Could you check a few things on this model? Use its own coordinates, in mm. Face numbers are marked on the shaded views. A direction names the side the tool comes from. Round coordinates to 2 decimals unless told otherwise and drop trailing zeros. Write each loop counter-clockwise with the first axis right and the second up, starting at its lowest first coordinate (ties: lowest second). Pieces come first, ordered by that corner, then holes. Notation, with made-up numbers: (68.5, -34) - (103.5, -34) arc R13 ccw to (103.5, -14) - close; hole circle Ø7 at (83.5, 16.5). An arc over 180 degrees is marked (long way). Put each result on its own line as item: value.
from build123d import *

# Parameters (mm, degrees)
SKETCH1_W           = 70
SKETCH1_H           = 55.65
BOSS_EXTRUDE1_DEPTH = 16.83
BOSS_EXTRUDE2_START = 16.83
SKETCH2_W           = 30.33
SKETCH2_H           = 30
BOSS_EXTRUDE2_DEPTH = 6.35
SKETCH3_R           = 14.055
BOSS_EXTRUDE3_DEPTH = 6.35
SKETCH4_R           = 14.055
CUT_EXTRUDE1_DEPTH  = 6.35
BOSS_EXTRUDE4_START = -35
SKETCH5_W           = 9.44
SKETCH5_H           = 4.86
BOSS_EXTRUDE4_DEPTH = 6.76
SKETCH6_R           = 1.7
BOSS_EXTRUDE5_DEPTH = 4
FILLET1_R           = 3
SKETCH7_R           = 7.14
BOSS_EXTRUDE6_DEPTH = 6.35
BOSS_EXTRUDE7_DEPTH = 4.35
FILLET3_R           = 3.5
CIRPATTERN11_COUNT  = 7
FILLET4_R           = 3.5


with BuildPart() as part:
    # Sketch1 → Boss-Extrude1 (new body)
    with BuildSketch(Plane(origin=(0, 0, 0), x_dir=(1, 0, 0), z_dir=(0, 1, 0))):
        Rectangle(SKETCH1_W, SKETCH1_H)
    extrude(amount=BOSS_EXTRUDE1_DEPTH)

    # Sketch2 → Boss-Extrude2 (add)
    with BuildSketch(Plane(origin=(0, 0, 0), x_dir=(1, 0, 0), z_dir=(0, 1, 0)).offset(BOSS_EXTRUDE2_START)):
        Rectangle(SKETCH2_W, SKETCH2_H)
    extrude(amount=BOSS_EXTRUDE2_DEPTH)

    # Sketch3 → Boss-Extrude3 (add)
    with BuildSketch(Plane(origin=(0, 23.18, 0), x_dir=(1, 0, 0), z_dir=(0, 1, 0))):
        Circle(SKETCH3_R)
    extrude(amount=-BOSS_EXTRUDE3_DEPTH)

    # Sketch4 → Cut-Extrude1 (cut)
    with BuildSketch(Plane(origin=(0, 23.18, 0), x_dir=(1, 0, 0), z_dir=(0, 1, 0))):
        with Locations(Location((0, 0, 0), (0, 0, 270))):
            Circle(SKETCH4_R)
    extrude(amount=-CUT_EXTRUDE1_DEPTH, mode=Mode.SUBTRACT)

    # Sketch5 → Boss-Extrude4 (add)
    with BuildSketch(Plane(origin=(0, 0, 0), x_dir=(0, 0, -1), z_dir=(1, 0, 0)).offset(BOSS_EXTRUDE4_START)):
        with Locations((18.775, 6.43)):
            Rectangle(SKETCH5_W, SKETCH5_H)
    extrude(amount=-BOSS_EXTRUDE4_DEPTH)

    # Sketch6 → Boss-Extrude5 (add)
    with BuildSketch(Plane(origin=(35, 0, 0), x_dir=(0, 0, -1), z_dir=(1, 0, 0))):
        with Locations(Location((-19.125364984, 11.29, 0), (0, 0, 180))):
            Circle(SKETCH6_R)
        with Locations(Location((-9.475364984, 11.29, 0), (0, 0, 180))):
            Circle(SKETCH6_R)
    extrude(amount=BOSS_EXTRUDE5_DEPTH)

    # Fillet1
    fillet1_edges = [part.edges().sort_by_distance(p)[0] for p in [
        (-35, 8.415, -27.825),
        (35, 8.415, -27.825),
        (35, 8.415, 27.825),
        (-35, 8.415, 27.825),
    ]]
    fillet(fillet1_edges, radius=FILLET1_R)

    # Sketch7 → Boss-Extrude6 (add)
    with BuildSketch(Plane(origin=(0, 16.83, 0), x_dir=(1, 0, 0), z_dir=(0, 1, 0))):
        with Locations(Location((0, 0, 0), (0, 0, 270))):
            Circle(SKETCH7_R)
    extrude(amount=BOSS_EXTRUDE6_DEPTH)

    # Sketch11 → Boss-Extrude7 (add)
    with BuildSketch(Plane(origin=(0, 16.83, 0), x_dir=(1, 0, 0), z_dir=(0, 1, 0))):
        with BuildLine():
            ThreePointArc((7.116145586, -0.583156929), (6.803943672, -2.164705639), (6.144899887, -3.635905029))
            ThreePointArc((6.144899887, -3.635905029), (11.187164412, -1.887909247), (13.51656418, 2.913529862))
            ThreePointArc((13.51656418, 2.913529862), (10.713284894, 0.438636341), (7.116145586, -0.583156929))
        make_face()
    boss_extrude7 = extrude(amount=BOSS_EXTRUDE7_DEPTH)

    # Fillet3
    # the kernel refuses this fillet: 3.5 mm, written as the material it takes off along each edge
    with BuildSketch(Plane(origin=(6.556014588, 21.18, -3.324644563), x_dir=(-0.9673093233437143, 0, 0.25359943409307006), z_dir=(-0.25359943409307006, 0, -0.9673093233437143))) as fillet3_piece_1_section:
        with BuildLine():
            CenterArc((6.972679966 - FILLET3_R, -FILLET3_R), FILLET3_R, 0, 90)
            Line((6.972679966 - FILLET3_R, 0), (6.972679966, 0))
            Line((6.972679966, 0), (6.972679966, -FILLET3_R))
        make_face()
    fillet3_piece_1 = revolve(axis=Axis((6.556014588, 21.18, -3.324644563), (0, 1, 0)), revolution_arc=233.858448906, mode=Mode.PRIVATE)
    fillet3_piece_1 = fillet3_piece_1 - Plane(origin=(0, 20.294110175, 0), x_dir=(0, 0, 1), z_dir=(0, -1, 0)) * Cylinder(7.14, 28, mode=Mode.PRIVATE)
    fillet3_piece_1 = fillet3_piece_1 - Plane(origin=(6.664387144, 20.294110175, -7.849834998), x_dir=(0.8113805957786566, 0, 0.5845182022776301), z_dir=(0, -1, 0)) * Cylinder(8.445083689, 28, mode=Mode.PRIVATE)
    add(fillet3_piece_1, mode=Mode.SUBTRACT)

    # CirPattern11: Boss-Extrude7 ×7 about axis
    cirpattern11_axis = Axis((0, 0, 0), (0, 1, 0))
    for i in range(1, CIRPATTERN11_COUNT):
        add(boss_extrude7.rotate(cirpattern11_axis, i * 360 / CIRPATTERN11_COUNT))

    # Fillet4
    # the kernel refuses this fillet: 3.5 mm, written as the material it takes off along each edge
    with BuildSketch(Plane(origin=(6.686920024, 21.18, 3.052816625), x_dir=(-0.8013795198577165, 0, -0.5981562213607877), z_dir=(0.5981562213607877, 0, -0.8013795198577165))) as fillet4_piece_1_section:
        with BuildLine():
            CenterArc((6.972679966 - FILLET4_R, -FILLET4_R), FILLET4_R, 0, 90)
            Line((6.972679966 - FILLET4_R, 0), (6.972679966, 0))
            Line((6.972679966, 0), (6.972679966, -FILLET4_R))
        make_face()
    fillet4_piece_1 = revolve(axis=Axis((6.686920024, 21.18, 3.052816625), (0, 1, 0)), revolution_arc=233.858448906, mode=Mode.PRIVATE)
    fillet4_piece_1 = fillet4_piece_1 - Plane(origin=(0, 20.294110175, 0), x_dir=(0, 0, 1), z_dir=(0, -1, 0)) * Cylinder(7.14, 28, mode=Mode.PRIVATE)
    fillet4_piece_1 = fillet4_piece_1 - Plane(origin=(10.292425554, 20.294110175, 0.316135614), x_dir=(0.04889279427778842, 0, 0.998804032164323), z_dir=(0, -1, 0)) * Cylinder(8.445083689, 28, mode=Mode.PRIVATE)
    add(fillet4_piece_1, mode=Mode.SUBTRACT)
    with BuildSketch(Plane(origin=(1.782438293, 21.18, 7.131444628), x_dir=(-0.0319945927557557, 0, -0.9994880419666827), z_dir=(0.9994880419666827, 0, -0.0319945927557557))) as fillet4_piece_2_section:
        with BuildLine():
            CenterArc((6.972679966 - FILLET4_R, -FILLET4_R), FILLET4_R, 0, 90)
            Line((6.972679966 - FILLET4_R, 0), (6.972679966, 0))
            Line((6.972679966, 0), (6.972679966, -FILLET4_R))
        make_face()
    fillet4_piece_2 = revolve(axis=Axis((1.782438293, 21.18, 7.131444628), (0, 1, 0)), revolution_arc=233.858448906, mode=Mode.PRIVATE)
    fillet4_piece_2 = fillet4_piece_2 & Plane(origin=(0, 20.294110175, 0), x_dir=(0, 0, 1), z_dir=(0, 1, 0)) * Cylinder(14.055, 28, mode=Mode.PRIVATE)
    fillet4_piece_2 = fillet4_piece_2 - Plane(origin=(0, 20.294110175, 0), x_dir=(0, 0, 1), z_dir=(0, -1, 0)) * Cylinder(7.14, 28, mode=Mode.PRIVATE)
    add(fillet4_piece_2, mode=Mode.SUBTRACT)
    with BuildSketch(Plane(origin=(-4.464255827, 21.18, 5.839949371), x_dir=(0.7614829152620437, 0, -0.6481849811311732), z_dir=(0.6481849811311732, 0, 0.7614829152620437))) as fillet4_piece_3_section:
        with BuildLine():
            CenterArc((6.972679966 - FILLET4_R, -FILLET4_R), FILLET4_R, 0, 90)
            Line((6.972679966 - FILLET4_R, 0), (6.972679966, 0))
            Line((6.972679966, 0), (6.972679966, -FILLET4_R))
        make_face()
    fillet4_piece_3 = revolve(axis=Axis((-4.464255827, 21.18, 5.839949371), (0, 1, 0)), revolution_arc=233.858448906, mode=Mode.PRIVATE)
    fillet4_piece_3 = fillet4_piece_3 & Plane(origin=(0, 20.294110175, 0), x_dir=(0, 0, 1), z_dir=(0, 1, 0)) * Cylinder(14.055, 28, mode=Mode.PRIVATE)
    fillet4_piece_3 = fillet4_piece_3 - Plane(origin=(0, 20.294110175, 0), x_dir=(0, 0, 1), z_dir=(0, -1, 0)) * Cylinder(7.14, 28, mode=Mode.PRIVATE)
    add(fillet4_piece_3, mode=Mode.SUBTRACT)
    with BuildSketch(Plane(origin=(-7.349274256, 21.18, 0.150853125), x_dir=(0.9815482566668393, 0, 0.19121459106011865), z_dir=(-0.19121459106011865, 0, 0.9815482566668393))) as fillet4_piece_4_section:
        with BuildLine():
            CenterArc((6.972679966 - FILLET4_R, -FILLET4_R), FILLET4_R, 0, 90)
            Line((6.972679966 - FILLET4_R, 0), (6.972679966, 0))
            Line((6.972679966, 0), (6.972679966, -FILLET4_R))
        make_face()
    fillet4_piece_4 = revolve(axis=Axis((-7.349274256, 21.18, 0.150853125), (0, 1, 0)), revolution_arc=233.858448906, mode=Mode.PRIVATE)
    fillet4_piece_4 = fillet4_piece_4 & Plane(origin=(0, 20.294110175, 0), x_dir=(0, 0, 1), z_dir=(0, 1, 0)) * Cylinder(14.055, 28, mode=Mode.PRIVATE)
    fillet4_piece_4 = fillet4_piece_4 - Plane(origin=(0, 20.294110175, 0), x_dir=(0, 0, 1), z_dir=(0, -1, 0)) * Cylinder(7.14, 28, mode=Mode.PRIVATE)
    add(fillet4_piece_4, mode=Mode.SUBTRACT)
    with BuildSketch(Plane(origin=(-4.700139271, 21.18, -5.651838602), x_dir=(0.4624877408659423, 0, 0.8866256761163174), z_dir=(-0.8866256761163174, 0, 0.4624877408659423))) as fillet4_piece_5_section:
        with BuildLine():
            CenterArc((6.972679966 - FILLET4_R, -FILLET4_R), FILLET4_R, 0, 90)
            Line((6.972679966 - FILLET4_R, 0), (6.972679966, 0))
            Line((6.972679966, 0), (6.972679966, -FILLET4_R))
        make_face()
    fillet4_piece_5 = revolve(axis=Axis((-4.700139271, 21.18, -5.651838602), (0, 1, 0)), revolution_arc=233.858448906, mode=Mode.PRIVATE)
    fillet4_piece_5 = fillet4_piece_5 & Plane(origin=(0, 20.294110175, 0), x_dir=(0, 0, 1), z_dir=(0, 1, 0)) * Cylinder(14.055, 28, mode=Mode.PRIVATE)
    fillet4_piece_5 = fillet4_piece_5 - Plane(origin=(0, 20.294110175, 0), x_dir=(0, 0, 1), z_dir=(0, -1, 0)) * Cylinder(7.14, 28, mode=Mode.PRIVATE)
    add(fillet4_piece_5, mode=Mode.SUBTRACT)
    with BuildSketch(Plane(origin=(1.488296449, 21.18, -7.198580584), x_dir=(-0.4048354768376397, 0, 0.9143895431891382), z_dir=(-0.9143895431891382, 0, -0.4048354768376397))) as fillet4_piece_6_section:
        with BuildLine():
            CenterArc((6.972679966 - FILLET4_R, -FILLET4_R), FILLET4_R, 0, 90)
            Line((6.972679966 - FILLET4_R, 0), (6.972679966, 0))
            Line((6.972679966, 0), (6.972679966, -FILLET4_R))
        make_face()
    fillet4_piece_6 = revolve(axis=Axis((1.488296449, 21.18, -7.198580584), (0, 1, 0)), revolution_arc=233.858448906, mode=Mode.PRIVATE)
    fillet4_piece_6 = fillet4_piece_6 & Plane(origin=(0, 20.294110175, 0), x_dir=(0, 0, 1), z_dir=(0, 1, 0)) * Cylinder(14.055, 28, mode=Mode.PRIVATE)
    fillet4_piece_6 = fillet4_piece_6 - Plane(origin=(0, 20.294110175, 0), x_dir=(0, 0, 1), z_dir=(0, -1, 0)) * Cylinder(7.14, 28, mode=Mode.PRIVATE)
    add(fillet4_piece_6, mode=Mode.SUBTRACT)


solid = part.part
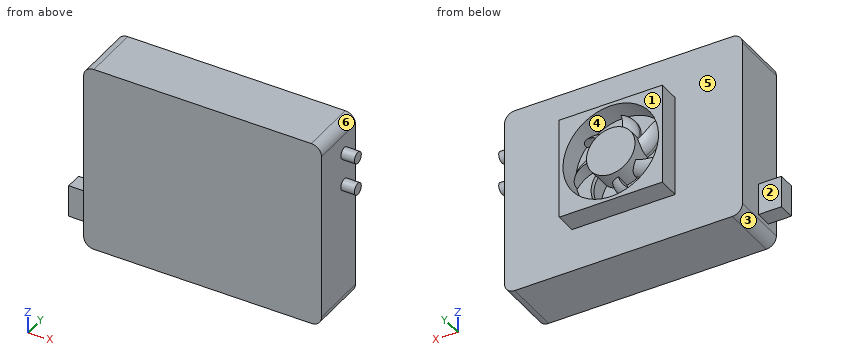
(1) Imagine slicing it at A-A, the plane y = 11.29. List the corners of the cut face in (x, z) for me (3 decimals).
Values found:
outline: (-35, -24.825) arc R3 ccw to (-32, -27.825) - (32, -27.825) arc R3 ccw to (35, -24.825) - (35, 7.775) - (39, 7.775) - (39, 11.175) - (35, 11.175) - (35, 17.425) - (39, 17.425) - (39, 20.825) - (35, 20.825) - (35, 24.825) arc R3 ccw to (32, 27.825) - (-32, 27.825) arc R3 ccw to (-35, 24.825) - close
(2) Please list where these lines run through material, in increasing order: probe 1 along X at (y, z) = (21.5, 0) (3 decimals); probe 2 along X at (y, z) = (19, -5.5) (3 decimals); probe 3 along Z at (x, y) = (-3.5, 21). Write a range as from..to.
Values found:
probe 1: x = -15.165..-14.055, -7.14..7.14, 14.055..15.165
probe 2: x = -15.165..-12.934, -10.975..4.553, 5.097..7.984, 12.934..15.165
probe 3: z = -15..-13.61, -6.22..6.22, 13.61..15
(3) I'm going to push flat-ended pins straight in: pin 1 (5.5 mm diameter, centred on x = -40, y = 6.5, fed in from -Z) (3 decimals); pin 2 (1.5 mm diameter, centred on x = 27, z = 14.5, fed in from +Y); pin 3 (8.5 mm diameter, centred on y = 8, z = -3, fed in from -X). Where does each tip first touch, or does it pass through?
Values found:
pin 1: stops at z = -23.495
pin 2: stops at y = 16.83
pin 3: stops at x = -35
(4) Imagine slicing it at B-B, the plane x = -34. List the corners of the cut face in (y, z) for me, then the cut area to 3 significant figures.
Values found:
outline: (0, -27.06) - (16.83, -27.06) - (16.83, 27.06) - (0, 27.06) - close
area: 911 mm^2
(5) For the marked faces 1 and 2, which set-ups out of +Z, -Z, +X, -X, +Y, -Y let a thin tool reach every point of the face, with its end or its side?
Values found:
face 1: +Z, -Z, +X, -X, +Y
face 2: +Z, -Z, -X, +Y
(6) If we mould it in two halves opening along Z, with no side actions, what happens to the marked faces 3, 4, 5 and 6? For each: pulls with the +Z half, pulls with the -Z half, needs draft (parallel to the pull), parting line crosses it, or undercut.
Values found:
face 3: pulls with the -Z half
face 4: undercut
face 5: needs draft
face 6: pulls with the +Z half
